```python
from build123d import *

# Parameters (mm, degrees)
SALIENTE_EXTRUIR1_DEPTH             = 24.75
CROQUIS2_W                          = 11
CROQUIS2_H                          = 3
CROQUIS3_R                          = 6
CORTAR_EXTRUIR1_DEPTH               = 46
CORTAR_EXTRUIR2_START               = -5
CROQUIS4_R                          = 16
CROQUIS4_R_2                        = 11
CORTAR_EXTRUIR2_DEPTH               = 5
TALADRO_ROSCADO_M61_D               = 5
TALADRO_ROSCADO_1_8_NPT1_AT_2_COUNT = 2
TALADRO_ROSCADO_1_8_NPT1_AT_2_PITCH = 31.5


with BuildPart() as part:
    # Croquis1 → Saliente-Extruir1 (new, symmetric)
    with BuildSketch(Plane.XY):
        Polygon((8, -23), (8, -25), (19.85, -25), (22, -22.85), (22, -9.15), (28, -7.5), (28, 7.5), (22, 9.15), (22, 22.85), (19.85, 25), (8, 25), (8, 23), (10, 23), (10, 22), (1, 22), (1, 25), (-1, 25), (-1, 22), (-10, 22), (-10, 23), (-8, 23), (-8, 25), (-19.85, 25), (-22, 22.85), (-22, 8), (-20, 8), (-20, 10), (-19, 10), (-19, 1), (-22, 1), (-22, -1), (-19, -1), (-19, -10), (-20, -10), (-20, -8), (-22, -8), (-22, -22.85), (-19.85, -25), (-8, -25), (-8, -23), (-10, -23), (-10, -22), (-1, -22), (-1, -25), (1, -25), (1, -22), (10, -22), (10, -23), align=None)
    extrude(amount=SALIENTE_EXTRUIR1_DEPTH, both=True)

    # Croquis2 → Revolución1 (revolve)
    with BuildSketch(Plane(origin=(0, 0, 0), x_dir=(1, 0, 0), z_dir=(0, 1, 0))):
        with Locations((5.5, 26.25)):
            Rectangle(CROQUIS2_W, CROQUIS2_H)
    revolve(axis=Axis((0, 0, -24.75), (0, 0, -1)))

    # Croquis3 → Cortar-Extruir1 (cut)
    with BuildSketch(Plane(origin=(0, 0, -27.75), x_dir=(-1, 0, 0), z_dir=(0, 0, -1))):
        Circle(CROQUIS3_R)
    extrude(amount=-CORTAR_EXTRUIR1_DEPTH, mode=Mode.SUBTRACT)

    # Croquis4 → Cortar-Extruir2 (cut)
    with BuildSketch(Plane(origin=(0, 0, -24.75), x_dir=(-1, 0, 0), z_dir=(0, 0, -1)).offset(CORTAR_EXTRUIR2_START)):
        Circle(CROQUIS4_R)
        with Locations(Location((0, 0, 0), (0, 0, 180))):
            Circle(CROQUIS4_R_2, mode=Mode.SUBTRACT)
    extrude(amount=CORTAR_EXTRUIR2_DEPTH, mode=Mode.SUBTRACT)

    # Taladro roscado M61 (through all)
    with Locations(Plane(origin=(0, 0, -24.75), x_dir=(-1, 0, 0), z_dir=(0, 0, -1))):
        with Locations((17, -17), (-17, -17), (-17, 17), (17, 17)):
            Hole(TALADRO_ROSCADO_M61_D / 2)

    # Croquis11 → Taladro roscado 1/8 NPT1 (revolve, cut)
    with BuildSketch(Plane(origin=(28, 0, -15.75), x_dir=(0, 0, -1), z_dir=(0, 1, 0))):
        Polygon((0, 0), (0, 14.153468714), (4.2164, 11.62), (4.2164, 6.92), (4.936178933, 6.92), (5.143373, 0), align=None)
    taladro_roscado_1_8_npt1 = revolve(axis=Axis((34.35, 0, -15.75), (-1, 0, 0)), mode=Mode.SUBTRACT)

    # Taladro roscado 1/8 NPT1 at 2: Taladro roscado 1/8 NPT1 ×2
    with Locations(*[(0, 0, i * TALADRO_ROSCADO_1_8_NPT1_AT_2_PITCH) for i in range(1, TALADRO_ROSCADO_1_8_NPT1_AT_2_COUNT)]):
        add(taladro_roscado_1_8_npt1, mode=Mode.SUBTRACT)


solid = part.part
```
For this review, take the finished solid that the model builds, in its own axes (mm). A direction names the side the tool comes from. Give positions to 0.01 mm unless a question says otherwise; leave off trailing zeros. Order: outer loops, then holes, each group sorted by start corner. A loop starts at its lowest first (then second) coordinate and runs counter-clockwise, first axis right, second up.
1) The part is to be moulded in two halves that separate along Y. For faces 1 (the face through (20.94, 23.91, 0.35)), 2 (the face through (-22, -15, 0)), 3 (the face through (-2.38, 10.74, -23.69)), say which applies: released by +Y, released by -Y, zero draft, split by the parting line, or undercut.
2) Wall thickness on line 1 (Z direction, x = 18, y = 0); line 2 (Y direction, x = 9, z = 16); line 3 (Y direction, x = 0, z = -21): over which ranges is each line inside the solid? List them lowest first.
3) Take a section at B-B (x = -17). Give the boundary of the cut face in (y, z).
4) For faces 4 (the face through (1, 23, 0)), 5 (the face through (21.08, 4, 18)), 6 (the face through (22, -16, 0)), 7 (the face through (-9, 23, 0)), list the 3-axis set-ups (+Z, -Z, +X, -X, +Y, -Y) from which the entire face can be reached by the end or side of a thin tool; tool diameter is ignored.
5) Take a section at A-A (y = 17). Give the boundary of the cut face in (x, z), then the cut area to 3 significant figures.
6) Insertion check: pin 1 (1.6 mm diameter, centred on y = -23.5, z = 9, fed in from +X); pin 2 (4 mm diameter, centred on x = 5, z = 9, fed in from -Y). Each pin has a flat end and moves straight along its axis. Give the tip position at first contact, or say it passes through.
7) Take a section at C-C (z = -1). State how many separate pieces and enclosed holes the cut face has, then the cut area to 3 significant figures.
8) Take a section at D-D (x = 0). Give the boundary of the cut face in (y, z).
Derived:
1. face 1: released by +Y
1. face 2: zero draft
1. face 3: undercut
2. line 1: z = -24.75 to -19.97, -11.53 to 11.53, 19.97 to 24.75
2. line 2: y = -25 to -23, -22 to 22, 23 to 25
2. line 3: y = -25 to -16, -11 to -6, 6 to 11, 16 to 25
3. outline: (-25, -24.75) - (-19.5, -24.75) - (-19.5, 24.75) - (-25, 24.75) - close; (-14.5, -24.75) - (14.5, -24.75) - (14.5, 24.75) - (-14.5, 24.75) - close; (19.5, -24.75) - (25, -24.75) - (25, 24.75) - (19.5, 24.75) - close
4. face 4: +Z, -Z, +Y
4. face 5: +X
4. face 6: +Z, -Z, +X, -Y
4. face 7: +Z, -Z
5. outline: (-22, -24.75) - (-19.5, -24.75) - (-19.5, 24.75) - (-22, 24.75) - close; (-14.5, -24.75) - (14.5, -24.75) - (14.5, 24.75) - (-14.5, 24.75) - close; (19.5, -24.75) - (22, -24.75) - (22, 24.75) - (19.5, 24.75) - close
5. area: 1,680 mm2
6. pin 1: stops at x = 22
6. pin 2: stops at y = -22
7. separate pieces: 1
7. enclosed holes: 5
7. area: 1,960 mm2
8. outline: (-25, -24.75) - (-16, -24.75) - (-16, -19.75) - (-11, -19.75) - (-11, -27.75) - (-6, -27.75) - (-6, 18.25) - (6, 18.25) - (6, -27.75) - (11, -27.75) - (11, -19.75) - (16, -19.75) - (16, -24.75) - (25, -24.75) - (25, 24.75) - (-25, 24.75) - close
